The model under review builds one solid part; all positions refer to its coordinate system, in mm. A direction names the side the tool comes from. Give positions to 0.01 mm unless a question says otherwise; leave off trailing zeros. Loops run counter-clockwise (first coordinate to the right, second up) from the corner with the lowest first, then second, coordinate; pieces in that order, holes last. Notation, with made-up numbers: (40, 86.5) - (91, 86.5) arc R25 ccw to (91, 100.5) - close; hole circle Ø5 at (64, 53). An arc over 180 degrees is marked (long way). Return JSON: item names as keys, results as strings. Group by question number.
```python
from build123d import *

# Parameters (mm, degrees)
SKETCH1_W           = 152.4
SKETCH1_H           = 152.4
BOSS_EXTRUDE1_DEPTH = 76.2
SKETCH4_R           = 25.4
CUT_EXTRUDE2_DEPTH  = 25.4
SKETCH5_R           = 25.4
BOSS_EXTRUDE2_DEPTH = 25.4
SKETCH6_W           = 127
SKETCH6_H           = 127
CUT_EXTRUDE3_DEPTH  = 12.7


with BuildPart() as part:
    # Sketch1 → Boss-Extrude1 (new, symmetric)
    with BuildSketch(Plane(origin=(0, 0, 0), x_dir=(1, 0, 0), z_dir=(0, 1, 0))):
        Rectangle(SKETCH1_W, SKETCH1_H)
    extrude(amount=BOSS_EXTRUDE1_DEPTH, both=True)

    # Sketch2 → Cut-Revolve1 (revolve, cut)
    with BuildSketch(Plane.XY, mode=Mode.PRIVATE) as cut_revolve1_sk:
        Polygon((0, 12.7), (13.97, 12.7), (13.97, 57.15), (33.02, 76.2), (0, 76.2), align=None)
    revolve(cut_revolve1_sk.sketch.rotate(Axis((0, 0, 0), (0, 1, 0)), 90), axis=Axis((0, 0, 0), (0, 1, 0)), mode=Mode.SUBTRACT)

    # Sketch4 → Cut-Extrude2 (cut)
    with BuildSketch(Plane.XY.offset(76.2)):
        Circle(SKETCH4_R)
    extrude(amount=-CUT_EXTRUDE2_DEPTH, mode=Mode.SUBTRACT)

    # Sketch5 → Boss-Extrude2 (add)
    with BuildSketch(Plane(origin=(0, 0, -76.2), x_dir=(-1, 0, 0), z_dir=(0, 0, -1))):
        with Locations(Location((0, 0, 0), (0, 0, 180))):
            Circle(SKETCH5_R)
    extrude(amount=BOSS_EXTRUDE2_DEPTH)

    # Sketch6 → Cut-Extrude3 (cut)
    with BuildSketch(Plane.ZY.offset(76.2)):
        Rectangle(SKETCH6_W, SKETCH6_H)
    extrude(amount=-CUT_EXTRUDE3_DEPTH, mode=Mode.SUBTRACT)


solid = part.part
```
1) For pin 1 Ø6 at (y, z) = (-16, -80.5) entering from +X; pin 2 Ø14 at (x, z) = (-4.5, -6) entering from +Y; pin 3 Ø10 at (y, z) = (26.5, 47.5) entering from -X, all flat-tipped, find the tip position at first contact; note any pin that passes through.
2) Draft analysis for pull direction X (two halves, no side actions). For faces 4 (the face through (-70, 63.5, -1)), 5 (the face through (-13.85, 35.24, 1.82)), 6 (the face through (76.2, 1, 1)), state which applies: +X half, -X half, draft (parallel to the pull), parting line (faces both ways), or undercut.
3) We need section B-B, the plane z = 48. Write out the cut boundary in (x, y), plus the area to 3 significant figures.
4) We need section C-C, the plane x = 0. Write out the cut boundary in (y, z).
5) We need section A-A, the plane y = 43.5. Write out the cut boundary in (x, z), plus the area to 3 significant figures.
6) Tool access review of faces 1 (the face through (-5.506, -24.796, 63.678)), 2 (the face through (-70, -1, -63.5)), 3 (the face through (11.721, 22.534, -88.722)): name each direction out of +Z, -Z, +X, -X, +Y, -Y from which nothing blocks a thin tool from reaching the whole face with its end or side.
7) We need section D-D, the plane y = 0. Write out the cut boundary in (x, z), plus the area to 3 significant figures.
8) To check wall thickness, follow line 1 (Z direction, x = -69, y = 58); line 2 (X direction, y = -47, z = 27.5); line 3 (Z direction, x = 65.5, y = 63). State the ranges of each line that lie inside material, in increasing order.
Findings:
{
 "1": {"pin 1": "stops at x = 21.82", "pin 2": "stops at y = 57.68", "pin 3": "stops at x = -63.5"},
 "2": {"face 4": "draft", "face 5": "undercut", "face 6": "+X half"},
 "3": {"outline": "(-76.2, -76.2) - (76.2, -76.2) - (76.2, 76.2) - (-76.2, 76.2) - (-76.2, 63.5) - (-63.5, 63.5) - (-63.5, -63.5) - (-76.2, -63.5) - close", "area": "21,600 mm^2"},
 "4": {"outline": "(-76.2, -76.2) - (-25.4, -76.2) - (-25.4, -101.6) - (25.4, -101.6) - (25.4, -76.2) - (76.2, -76.2) - (76.2, -33.02) - (57.15, -13.97) - (12.7, -13.97) - (12.7, 13.97) - (57.15, 13.97) - (76.2, 33.02) - (76.2, 76.2) - (25.4, 76.2) - (25.4, 50.8) - (-25.4, 50.8) - (-25.4, 76.2) - (-76.2, 76.2) - close"},
 "5": {"outline": "(-76.2, -76.2) - (76.2, -76.2) - (76.2, 76.2) - (-76.2, 76.2) - (-76.2, 63.5) - (-63.5, 63.5) - (-63.5, -63.5) - (-76.2, -63.5) - close; hole circle Ø27.94 at (0, 0)", "area": "21,000 mm^2"},
 "6": {"face 1": "+Z", "face 2": "-X", "face 3": "-Z"},
 "7": {"outline": "(-76.2, -76.2) - (-25.4, -76.2) - (-25.4, -101.6) - (25.4, -101.6) - (25.4, -76.2) - (76.2, -76.2) - (76.2, 76.2) - (25.4, 76.2) - (25.4, 50.8) - (-25.4, 50.8) - (-25.4, 76.2) - (-76.2, 76.2) - (-76.2, 63.5) - (-63.5, 63.5) - (-63.5, -63.5) - (-76.2, -63.5) - close", "area": "21,600 mm^2"},
 "8": {"line 1": "z = -76.2 to -63.5, 63.5 to 76.2", "line 2": "x = -63.5 to 76.2", "line 3": "z = -76.2 to 76.2"}
}
